Autodesk Inventor part; units mm, degrees
ref_plane "YZ Plane" through (0, 0, 0) normal (1, 0, 0) x (0, 1, 0)
ref_plane "XZ Plane" through (0, 0, 0) normal (0, 1, 0) x (-1, 0, 0)
ref_plane "XY Plane" through (0, 0, 0) normal (0, 0, 1) x (1, 0, 0)
sketch "Sketch1" plane through (0, 0, 0) normal (0, 0, 1) x (1, 0, 0)
  circle A0 centre (0, 0) radius 90
  circle A1 centre (0, 8) radius 1.65
  circle A2 centre (-8, 0) radius 1.65
  circle A3 centre (0, -8) radius 1.65
  circle A4 centre (8, 0) radius 1.65
  dimension "d0" = 180
  dimension "d1" = 3.3
  dimension "d2" = 8
  dimension "d5" = 360
extrude "Extrusion1" add sketch "Sketch1" along normal blind 3.5
equation "\"BendRadius\" = Thickness"
equation "\"BendReliefWidth\" = Thickness"
equation "\"BendReliefDepth\" = 0.5 * Thickness"
equation "\"CornerReliefSize\" = 4 * Thickness"
equation "\"MinimumRemnant\" = 2 * Thickness"
equation "\"TransitionRadius\" = BendRadius"
equation "\"JacobiRadiusSize\" = BendRadius"
equation "\"GapSize\" = Thickness"
properties part number "bàn xoay"
Source: CAD feature listing. Evaluate the final solid. Frame: model axes, mm. Coordinates: 2 decimals unless noted, no trailing zeros. Loops run counter-clockwise (first coordinate to the right, second up) from the corner with the lowest first, then second, coordinate; pieces in that order, holes last. Notation, with made-up numbers: (-1.75, 53) -> (13.25, 53) arc R26 cw to (13.25, 87) -> close; hole circle Ø3 at (-22.75, -37). An arc over 180 degrees is marked (long way). Answer in a Markdown table with one row per item. Add a question column.
Q1. Section B-B on x = -54. Return the cut outline in (y, z), and give its area (3 significant figures).
Q2. Section C-C on y = 62. Return the cut outline in (x, z).
Q3. Ray query, line 1 along Y through (x, z) = (0, 2.85); line 2 along Y through (x, z) = (1.5, 1.7); line 3 along Y through (x, z) = (-8, 1.8). Return the intervals inside material, ascending.
Q4. Section A-A on z = 1.75. Return the cut outline in (x, y), and give its area (3 significant figures).
Q5. Contact query for flat-ended pins moving along their axis: pin 1 Ø3 at (x, y) = (0, 8) entering from -Z; pin 2 Ø1.5 at (x, z) = (70.5, 3) entering from -Y; pin 3 Ø1.5 at (y, z) = (36, 0.5) entering from -X. Output: stop coordinate, or through.
Computed values:
| question | item | result |
|---|---|---|
| 1 | outline | (-72, 0) -> (72, 0) -> (72, 3.5) -> (-72, 3.5) -> close |
| 1 | area | 504 mm^2 |
| 2 | outline | (-65.24, 0) -> (65.24, 0) -> (65.24, 3.5) -> (-65.24, 3.5) -> close |
| 3 | line 1 | y = -90 to -9.65, -6.35 to 6.35, 9.65 to 90 |
| 3 | line 2 | y = -89.99 to -8.69, -7.31 to 7.31, 8.69 to 89.99 |
| 3 | line 3 | y = -89.64 to -1.65, 1.65 to 89.64 |
| 4 | outline | circle Ø180 at (0, 0); hole circle Ø3.3 at (-8, 0); hole circle Ø3.3 at (0, -8); hole circle Ø3.3 at (0, 8); hole circle Ø3.3 at (8, 0) |
| 4 | area | 25,400 mm^2 |
| 5 | pin 1 | passes through |
| 5 | pin 2 | stops at y = -56.88 |
| 5 | pin 3 | stops at x = -82.81 |
